Could you check a few things on this model? Use its own coordinates, in mm. A direction names the side the tool comes from. Give positions to 0.01 mm unless a question says otherwise; leave off trailing zeros. Order: outer loops, then holes, each group sorted by start corner. A loop starts at its lowest first (then second) coordinate and runs counter-clockwise, first axis right, second up. Notation, with made-up numbers: M -16,-28 L 10,-28 A13 ccw 10,-3 Z; hole C 82.25,37 d10. An arc over 180 degrees is marked long. Return JSON: item names as keys, results as strings. Group by question number.
```python
from build123d import *

# Parameters (mm, degrees)
CORTAR_EXTRUIR1_REACH     = 21.1
CROQUIS2_R                = 1.25
TALADRO_ROSCADO_M31_D     = 2.5
TALADRO_ROSCADO_M31_DEPTH = 8.5
TALADRO_ROSCADO_M31_TIP   = 0.751075774


with BuildPart() as part:
    # Croquis1 → Revolución1 (revolve)
    with BuildSketch(Plane.XY):
        Polygon((6.35, 0), (6.35, 15.1), (10.15, 15.1), (10.15, 19.1), (3.25, 19.1), (3.25, 0), align=None)
    revolve(axis=Axis((0, 0, 0), (0, 1, 0)))

    # Croquis2 → Cortar-Extruir1 (cut, up to next)
    with BuildSketch(Plane(origin=(0, 19.1, 0), x_dir=(1, 0, 0), z_dir=(0, 1, 0)), mode=Mode.PRIVATE) as cortar_extruir1_sk1:
        with Locations((6.9715045, -4.025)):
            Circle(CROQUIS2_R)
    cortar_extruir1_tool1 = extrude(cortar_extruir1_sk1.sketch, amount=-CORTAR_EXTRUIR1_REACH, mode=Mode.PRIVATE) & part.part
    add(cortar_extruir1_tool1.solids().sort_by_distance((6.971505, 19.1, 4.025))[0], mode=Mode.SUBTRACT)
    # Croquis2 → Cortar-Extruir1 (cut, up to next)
    with BuildSketch(Plane(origin=(0, 19.1, 0), x_dir=(1, 0, 0), z_dir=(0, 1, 0)), mode=Mode.PRIVATE) as cortar_extruir1_sk2:
        with Locations((0, 8.05)):
            Circle(CROQUIS2_R)
    cortar_extruir1_tool2 = extrude(cortar_extruir1_sk2.sketch, amount=-CORTAR_EXTRUIR1_REACH, mode=Mode.PRIVATE) & part.part
    add(cortar_extruir1_tool2.solids().sort_by_distance((0, 19.1, -8.05))[0], mode=Mode.SUBTRACT)
    # Croquis2 → Cortar-Extruir1 (cut, up to next)
    with BuildSketch(Plane(origin=(0, 19.1, 0), x_dir=(1, 0, 0), z_dir=(0, 1, 0)), mode=Mode.PRIVATE) as cortar_extruir1_sk3:
        with Locations((-6.9715045, -4.025)):
            Circle(CROQUIS2_R)
    cortar_extruir1_tool3 = extrude(cortar_extruir1_sk3.sketch, amount=-CORTAR_EXTRUIR1_REACH, mode=Mode.PRIVATE) & part.part
    add(cortar_extruir1_tool3.solids().sort_by_distance((-6.971505, 19.1, 4.025))[0], mode=Mode.SUBTRACT)

    # Taladro roscado M31
    with Locations(Plane(origin=(0, 15.1, -8.05), x_dir=(0, 0, -1), z_dir=(0, -1, 0))):
        with Locations((0, 0), (-12.075, 6.9715045), (-12.075, -6.9715045)):
            Hole(TALADRO_ROSCADO_M31_D / 2, depth=TALADRO_ROSCADO_M31_DEPTH)
            with Locations((0, 0, -(TALADRO_ROSCADO_M31_DEPTH + TALADRO_ROSCADO_M31_TIP / 2))):  # 118° drill point
                Cone(0, TALADRO_ROSCADO_M31_D / 2, TALADRO_ROSCADO_M31_TIP, mode=Mode.SUBTRACT)


solid = part.part
```
1. I need wall thicknesses on L1, parallel to Z at x = 0, y = 11.25; L2, parallel to X at y = 16, z = -8.05. Which ranges of each line are inside material? Lowest first, please. Write a range as from..to.
2. Which directions (+Z, -Z, +X, -X, +Y, -Y) give clear straight access to the entire face, cutting with the end or side of a thin tool? Please do faces 4 (the flat face through (0, 19.1, 4)), 5 (the flat face through (0, 15.1, 7)).
3. If we mould it in two halves opening along X, with no side actions, what happens to faces 1 (the cylindrical face through (-7.96, 17.13, 4.79)), 2 (the flat face through (3, 0, -2)), 3 (the cylindrical face through (-8.05, 17.13, 6.18))? For each: pulls with the +X half, pulls with the -X half, needs draft (parallel to the pull), parting line crosses it, or undercut.
4. Imagine slicing it at C-C, the plane y = 5.5. Please give me the cut outline in (x, z).
5. For pin 1 (1.5 mm diameter, centred on y = 13, z = 0.5, fed in from +X); pin 2 (8.5 mm diameter, centred on x = 0, z = 0, fed in from +Y); pin 3 (3 mm diameter, centred on x = -4.5, y = 13.5, fed in from +Z); pin 4 (3 mm diameter, centred on x = -6.97, z = 4.03, fed in from -Y), each with a flat end and sliding along its axis, tell me the tip position at first contact or that it passes through.
6. Imagine slicing it at D-D, the plane x = 4.25. Please give me the cut outline in (y, z), plus the area to 3 significant figures.
7. Imagine slicing it at B-B, the plane x = -2.25. Please give me the cut outline in (y, z).
8. Imagine slicing it at A-A, the plane z = 0. Please give me the cut outline in (x, y).
Values:
{
 "1": {"L1": "z = -6.35..-3.25, 3.25..6.35", "L2": "x = -6.18..-1.25, 1.25..6.18"},
 "2": {"face 4": "+Z, -Z, +X, -X, +Y", "face 5": "-Y"},
 "3": {"face 1": "undercut", "face 2": "needs draft", "face 3": "parting line crosses it"},
 "4": {"outline": "C 0,0 d12.7; hole C 0,0 d6.5"},
 "5": {"pin 1": "stops at x = 6.35", "pin 2": "stops at y = 19.1", "pin 3": "stops at z = 5.6", "pin 4": "stops at y = 15.1"},
 "6": {"outline": "M 0,-4.72 L 15.1,-4.72 L 15.1,-9.22 L 19.1,-9.22 L 19.1,9.22 L 15.1,9.22 L 15.1,4.72 L 0,4.72 Z", "area": "216 mm²"},
 "7": {"outline": "M 0,-5.94 L 15.1,-5.94 L 15.1,-9.9 L 19.1,-9.9 L 19.1,-2.35 L 0,-2.35 Z; M 0,2.35 L 19.1,2.35 L 19.1,9.9 L 15.1,9.9 L 15.1,5.94 L 0,5.94 Z"},
 "8": {"outline": "M -10.15,15.1 L -6.35,15.1 L -6.35,0 L -3.25,0 L -3.25,19.1 L -10.15,19.1 Z; M 3.25,0 L 6.35,0 L 6.35,15.1 L 10.15,15.1 L 10.15,19.1 L 3.25,19.1 Z"}
}
